from build123d import *

# Parameters (mm, degrees)
SKETCH1_W           = 120
SKETCH1_H           = 80
SKETCH1_R           = 1.6
SKETCH1_R_2         = 3
BOSS_EXTRUDE1_DEPTH = 4
FILLET1_R           = 2
FILLET2_R           = 2
FILLET3_R           = 2
FILLET4_R           = 2


with BuildPart() as part:
    # Sketch1 → Boss-Extrude1 (new body)
    with BuildSketch(Plane(origin=(0, 0, 0), x_dir=(1, 0, 0), z_dir=(0, 1, 0))):
        with Locations((60, 40)):
            Rectangle(SKETCH1_W, SKETCH1_H)
        with Locations((3, 77)):
            Circle(SKETCH1_R, mode=Mode.SUBTRACT)
        with Locations((3, 3)):
            Circle(SKETCH1_R, mode=Mode.SUBTRACT)
        with Locations((117, 77)):
            Circle(SKETCH1_R, mode=Mode.SUBTRACT)
        with Locations((117, 3)):
            Circle(SKETCH1_R, mode=Mode.SUBTRACT)
        with Locations((60, 75)):
            Circle(SKETCH1_R_2, mode=Mode.SUBTRACT)
    extrude(amount=BOSS_EXTRUDE1_DEPTH)

    # Fillet1
    fillet1_edges = [part.edges().sort_by_distance(p)[0] for p in [
        (0, 2, 0),
    ]]
    fillet(fillet1_edges, radius=FILLET1_R)

    # Fillet2
    fillet2_edges = [part.edges().sort_by_distance(p)[0] for p in [
        (120, 2, 0),
    ]]
    fillet(fillet2_edges, radius=FILLET2_R)

    # Fillet3
    fillet3_edges = [part.edges().sort_by_distance(p)[0] for p in [
        (120, 2, -80),
    ]]
    fillet(fillet3_edges, radius=FILLET3_R)

    # Fillet4
    fillet4_edges = [part.edges().sort_by_distance(p)[0] for p in [
        (0, 2, -80),
    ]]
    fillet(fillet4_edges, radius=FILLET4_R)


solid = part.part
CAD build for the part. Positions are in the model's coordinates, mm. Coordinates: 2 decimals unless noted, no trailing zeros. Loops run counter-clockwise (first coordinate to the right, second up) from the corner with the lowest first, then second, coordinate; pieces in that order, holes last. Notation, with made-up numbers: (39.25, 41) - (66.25, 41) arc R32 ccw to (66.25, 78) - close; hole circle Ø6 at (11.5, 63.5). An arc over 180 degrees is marked (long way). Write item = value, one per line. Start each with the question number.
Q1. Flat gauge pin, fed straight in: pin 1 Ø2.5 at (x, z) = (3, -77) entering from +Y. Where does the tip first touch, or does it go through?
Q2. Pull direction Z, two halves, no side cores. Call faces 1 (the flat face through (59, 2, -80)), 2 (the flat face through (120, 2, -39)), 3 (the cylindrical face through (118.526, 1.972, -3.481)): pulls with the +Z half, pulls with the -Z half, needs draft (parallel to the pull), parting line crosses it, or undercut.
Q3. Drill centre lines: L1, parallel to X at y = 1.75, z = -3; L2, parallel to Z at x = 117, y = 1.85; L3, parallel to Z at x = 60, y = 2.45. Where is each one in solid material? Low to high.
Q4. Cut at A-A, the plane x = 60. List the corners of the cut face in (y, z), then the cut area to 3 significant figures.
Computed:
q1.pin_1 = through
q2.face_1 = pulls with the -Z half
q2.face_2 = needs draft
q2.face_3 = undercut
q3.L1 = 0 to 1.4, 4.6 to 115.4, 118.6 to 120
q3.L2 = -80 to -78.6, -75.4 to -4.6, -1.4 to 0
q3.L3 = -80 to -78, -72 to 0
q4.outline = (0, -80) - (4, -80) - (4, -78) - (0, -78) - close; (0, -72) - (4, -72) - (4, 0) - (0, 0) - close
q4.area = 296 mm²
